For this review, take the finished solid that the model builds, in its own axes (mm). A direction names the side the tool comes from. Round coordinates to 2 decimals unless told otherwise and drop trailing zeros. Loops run counter-clockwise (first coordinate to the right, second up) from the corner with the lowest first, then second, coordinate; pieces in that order, holes last.
```python
from build123d import *

# Parameters (mm, degrees)
F1_DEPTH = 6
F3_DEPTH = 4
F5_DEPTH = 2


with BuildPart() as f1:
    # F0 (on Front) → F1 (new body)
    with BuildSketch(Plane.XZ):
        with BuildLine():
            Line((0.5280444536, 6.5949463177), (0.2280896806, 6.6083750402))
            ThreePointArc((0.2280896806, 6.6083750402), (-4.4587573432, 4.7555534352), (-6.412563722, 0.1098970168))
            Line((-6.412563722, 0.1098970168), (-1.912563722, 0.1098970168))
            ThreePointArc((-1.912563722, 0.1098970168), (0.087436278, 2.1098970168), (2.087436278, 0.1098970168))
            Line((2.087436278, 0.1098970168), (6.587436278, 0.1098970168))
            ThreePointArc((6.587436278, 0.1098970168), (4.8368548288, 4.5475792304), (0.5280444536, 6.5949463177))
        make_face()
        with BuildLine():
            ThreePointArc((0.5280444536, 6.5949463177), (0.3781446168, 6.6033928905), (0.2280896806, 6.6083750402))
            Line((0.2280896806, 6.6083750402), (0.5280444536, 6.5949463177))
        make_face()
        with BuildLine():
            Line((-1.912563722, 0.1098970168), (-6.412563722, 0.1098970168))
            ThreePointArc((-6.412563722, 0.1098970168), (-4.6032413883, -4.3898299783), (-0.1825504819, -6.3844934203))
            Line((-0.1825504819, -6.3844934203), (0.92817218, -6.3355015856))
            ThreePointArc((0.92817218, -6.3355015856), (4.9718391772, -4.1787634173), (6.587436278, 0.1098970168))
            Line((6.587436278, 0.1098970168), (2.087436278, 0.1098970168))
            ThreePointArc((2.087436278, 0.1098970168), (0.087436278, -1.8901029832), (-1.912563722, 0.1098970168))
        make_face()
        with BuildLine():
            Line((33.8110580771, 5.1048938427), (0.5280444536, 6.5949463177))
            ThreePointArc((0.5280444536, 6.5949463177), (4.8368548288, 4.5475792304), (6.587436278, 0.1098970168))
            Line((6.587436278, 0.1098970168), (28.587436278, 0.1098970168))
            ThreePointArc((28.587436278, 0.1098970168), (30.1318689581, 3.7236283983), (33.8110580771, 5.1048938427))
        make_face()
        with BuildLine():
            Line((0.92817218, -6.3355015856), (-0.1825504819, -6.3844934203))
            ThreePointArc((-0.1825504819, -6.3844934203), (0.3738602571, -6.3837892479), (0.92817218, -6.3355015856))
        make_face()
        with BuildLine():
            Line((28.587436278, 0.1098970168), (6.587436278, 0.1098970168))
            ThreePointArc((6.587436278, 0.1098970168), (4.9718391772, -4.1787634173), (0.92817218, -6.3355015856))
            Line((0.92817218, -6.3355015856), (33.8077624157, -4.8852462637))
            ThreePointArc((33.8077624157, -4.8852462637), (30.1306770073, -3.5026942062), (28.587436278, 0.1098970168))
        make_face()
        with BuildLine():
            ThreePointArc((38.587436278, 0.1098970168), (37.2011676595, 3.5654643367), (33.8110580771, 5.1048938427))
            ThreePointArc((33.8110580771, 5.1048938427), (30.1318689581, 3.7236283983), (28.587436278, 0.1098970168))
            Line((28.587436278, 0.1098970168), (32.087436278, 0.1098970168))
            ThreePointArc((32.087436278, 0.1098970168), (33.587436278, 1.6098970168), (35.087436278, 0.1098970168))
            Line((35.087436278, 0.1098970168), (38.587436278, 0.1098970168))
        make_face()
        with BuildLine():
            Line((32.087436278, 0.1098970168), (28.587436278, 0.1098970168))
            ThreePointArc((28.587436278, 0.1098970168), (30.1306770073, -3.5026942062), (33.8077624157, -4.8852462637))
            ThreePointArc((33.8077624157, -4.8852462637), (37.200027501, -3.3468622539), (38.587436278, 0.1098970168))
            Line((38.587436278, 0.1098970168), (35.087436278, 0.1098970168))
            ThreePointArc((35.087436278, 0.1098970168), (33.587436278, -1.3901029832), (32.087436278, 0.1098970168))
        make_face()
    extrude(amount=F1_DEPTH)

    # F2 (on Front) → F3 (cut)
    with BuildSketch(Plane.XZ):
        with BuildLine():
            Line((2.8225806452, 0), (4.5, 0))
            ThreePointArc((4.5, 0), (4.0590400899, 1.9427283774), (2.8225806452, 3.5047166079))
            Line((2.8225806452, 3.5047166079), (2.8225806452, 0))
        make_face()
        with BuildLine():
            Line((13.5, 0), (4.5, 0))
            ThreePointArc((4.5, 0), (4.0590400899, -1.9427283774), (2.8225806452, -3.5047166079))
            Line((2.8225806452, -3.5047166079), (15.7336008924, -1.9863108073))
            ThreePointArc((15.7336008924, -1.9863108073), (14.1709405177, -1.4945236339), (13.5, 0))
        make_face()
        with BuildLine():
            ThreePointArc((2.8225806452, -3.5047166079), (4.0590400899, -1.9427283774), (4.5, 0))
            Line((4.5, 0), (2.8225806452, 0))
            Line((2.8225806452, 0), (2.8225806452, -3.5047166079))
        make_face()
        with BuildLine():
            ThreePointArc((2.8225806452, 3.5047166079), (4.0590400899, 1.9427283774), (4.5, 0))
            Line((4.5, 0), (13.5, 0))
            ThreePointArc((13.5, 0), (14.1709405177, 1.4945236339), (15.7336008924, 1.9863108073))
            Line((15.7336008924, 1.9863108073), (2.8225806452, 3.5047166079))
        make_face()
        with BuildLine():
            Line((2.8225806452, 0), (2.8225806452, 3.5047166079))
            ThreePointArc((2.8225806452, 3.5047166079), (1.496458363, 4.2438911824), (0, 4.5))
            Line((0, 4.5), (0, 0))
            Line((0, 0), (2.8225806452, 0))
        make_face()
        with BuildLine():
            ThreePointArc((0, -4.5), (1.496458363, -4.2438911824), (2.8225806452, -3.5047166079))
            Line((2.8225806452, -3.5047166079), (2.8225806452, 0))
            Line((2.8225806452, 0), (0, 0))
            Line((0, 0), (0, -4.5))
        make_face()
        with BuildLine():
            ThreePointArc((15.7336008924, 1.9863108073), (14.1709405177, 1.4945236339), (13.5, 0))
            ThreePointArc((13.5, 0), (14.1709405177, -1.4945236339), (15.7336008924, -1.9863108073))
            ThreePointArc((15.7336008924, -1.9863108073), (16.9945236339, -1.3290594823), (17.5, 0))
            ThreePointArc((17.5, 0), (16.9945236339, 1.3290594823), (15.7336008924, 1.9863108073))
        make_face()
        with BuildLine():
            Line((0, 0), (0, 4.5))
            ThreePointArc((0, 4.5), (-3.1819805153, 3.1819805153), (-4.5, 0))
            Line((-4.5, 0), (0, 0))
        make_face()
        with BuildLine():
            ThreePointArc((-4.5, 0), (-3.1819805153, -3.1819805153), (0, -4.5))
            Line((0, -4.5), (0, 0))
            Line((0, 0), (-4.5, 0))
        make_face()
    extrude(amount=F3_DEPTH, mode=Mode.SUBTRACT)

    # F4 (on face) → F5 (cut)
    with BuildSketch(Plane(origin=(0, 0, 0), x_dir=(-1, 0, 0), z_dir=(0, 1, 0))):
        with BuildLine():
            ThreePointArc((-16.0594756914, -3.4959212069), (-19.2027878035, -0.0038572282), (-15.9837236084, 3.418502714))
            Line((-15.9837236084, 3.418502714), (-32.5201968963, 2.8216355423))
            ThreePointArc((-32.5201968963, 2.8216355423), (-31.2720018674, 0.0697774052), (-32.4186347425, -2.7259241324))
            Line((-32.4186347425, -2.7259241324), (-16.0594756914, -3.4959212069))
        make_face()
    extrude(amount=-F5_DEPTH, mode=Mode.SUBTRACT)


solid = f1.part
```
(1) Add section B-B (z = -0.75). Give the boundary of the cut face in (x, y).
(2) Insertion check: pin 1 Ø3 at (y, z) = (-4.5, -3.5) entering from +X; pin 2 Ø1.5 at (y, z) = (-5, 2) entering from -X; pin 3 Ø1.5 at (x, z) = (28.5, 2) entering from +Y. Each pin has a flat end and moves straight along its axis. Give the tip position at first contact, or say it passes through.
(3) The part is to be moulded in two halves that separate along X. For faces 3 (the flat face through (17.4, -2.96, 5.84)), 4 (the cylindrical face through (32.397, -2.958, 1.023)), 5 (the flat face through (16, -6, 0)), say which applies: pulls with the +X half, pulls with the -X half, needs draft (parallel to the pull), parting line crosses it, or undercut.
(4) For L1, parallel to X at y = -2.85, z = -0.25; L2, parallel to X at y = -4.8, z = 0.75; L3, parallel to Z at x = 7.5, y = -3.3, list the stretches that pass through material, from the lowest coordinate up.
(5) Add section C-C (y = -1.15). Give the boundary of the cut face in (x, z), plus the area to 3 significant figures.
(6) Add section A-A (y = -5.4). Give the boundary of the cut face in (x, z).
(7) Add section D-D (x = 34.5). Give the boundary of the cut face in (y, z), plus the area to 3 significant figures.
(8) For faces 1 (the flat face through (9.188, -1.972, -2.756)), 2 (the cylindrical face through (1.995, -4.986, -0.491)), list the 3-axis set-ups (+Z, -Z, +X, -X, +Y, -Y) from which the entire face can be reached by the end or side of a thin tool; tool diameter is ignored.
Outcome:
1. outline: (-6.36, -6) - (-1.72, -6) - (-1.72, -4) - (-4.44, -4) - (-4.44, 0) - (-6.36, 0) - close; (1.89, -6) - (32.36, -6) - (32.36, 0) - (31.35, 0) - (31.35, -2) - (19.13, -2) - (19.13, 0) - (17.35, 0) - (17.35, -4) - (1.89, -4) - close; (34.82, -6) - (38.51, -6) - (38.51, 0) - (34.82, 0) - close
2. pin 1: stops at x = 38.12
2. pin 2: stops at x = -6.31
2. pin 3: stops at y = -2
3. face 3: pulls with the +X half
3. face 4: undercut
3. face 5: needs draft
4. L1: x = -6.4 to -4.49, 17.48 to 32.13, 35.04 to 38.57
4. L2: x = -6.38 to -1.81, 1.98 to 32.23, 34.94 to 38.55
4. L3: z = -6.05 to -2.95, 2.95 to 6.28
5. outline: (0.53, 6.59) arc R6.5 ccw (long way) to (0.93, -6.34) - (33.81, -4.89) arc R5 ccw to (33.81, 5.1) - close; hole (2.82, -3.5) - (15.73, -1.99) arc R2 ccw to (15.73, 1.99) - (2.82, 3.5) arc R4.5 ccw (long way) to start; hole (15.98, 3.42) arc R3.47 cw to (16.06, -3.5) - (32.42, -2.73) arc R3.81 cw to (32.52, 2.82) - close; hole circle Ø3 at (33.59, 0.11)
5. area: 271 mm2
6. outline: (0.53, 6.59) arc R6.5 ccw (long way) to (0.93, -6.34) - (33.81, -4.89) arc R5 ccw to (33.81, 5.1) - close; hole circle Ø4 at (0.09, 0.11); hole circle Ø3 at (33.59, 0.11)
7. outline: (-6, -4.81) - (0, -4.81) - (0, -1.08) - (-6, -1.08) - close; (-6, 1.3) - (0, 1.3) - (0, 5.03) - (-6, 5.03) - close
7. area: 44.7 mm2
8. face 1: +Y
8. face 2: +Y, -Y
